Design review of the part built by this model. Coordinates are the model's own, in mm. A direction names the side the tool comes from. Coordinates: 2 decimals unless noted, no trailing zeros. Write each loop counter-clockwise with the first axis right and the second up, starting at its lowest first coordinate (ties: lowest second). Pieces come first, ordered by that corner, then holes. Notation, with made-up numbers: M -10,23.5 L 8,23.5 A26 ccw 8,39.5 Z; hole C -27,-4 d2. An arc over 180 degrees is marked long. Write item = value, one per line.
Autodesk Inventor part; units mm, degrees
ref_plane "YZ Plane" through (0, 0, 0) normal (1, 0, 0) x (0, 1, 0)
ref_plane "XZ Plane" through (0, 0, 0) normal (0, 1, 0) x (-1, 0, 0)
ref_plane "XY Plane" through (0, 0, 0) normal (0, 0, 1) x (1, 0, 0)
sketch "Sketch1" plane through (0, 0, 0) normal (0, 0, 1) x (1, 0, 0)
  circle A0 centre (0, 0) radius 24.5
  dimension "d0" = 49
extrude "Extrusion1" add sketch "Sketch1" along normal blind 83
sketch "Sketch2" plane through (0, 0, 0) normal (0, 0, 1) x (1, 0, 0)
  circle A0 centre (0, 0) radius 3
  dimension "d3" = 6
extrude "Extrusion2" add sketch "Sketch2" against normal blind 20
chamfer "Chamfer1" distance 3 distance2 8 1 edges at (-24.5, 0, 0) measured on face at (17.067, -2.1937, 0)
sketch "Sketch4" plane through (0, 0, 83) normal (0, 0, 1) x (1, 0, 0)
  circle A0 centre (0, 0) radius 7.25
  circle A1 centre (0, 0) radius 24.5
  dimension "d10" = 14.5
extrude "Extrusion3" cut sketch "Sketch4" against normal blind 5
chamfer "Chamfer2" distance 8.41 angle 45 1 edges at (-24.5, 0, 78)
properties part number "Motor SK3 5065 275KV"
Q1. For P1, Ø1, axis at x = -8.5, z = 72.5, coming from the +Y side; P2, Ø6, axis at y = 15.5, z = 52.5, coming from the +X side; P3, Ø1, axis at x = 16.5, z = 21, coming from the +Y side; P4, Ø16, axis at x = -7.5, y = -6.5, coming from the +Z side, all flat-tipped, find the tip position at first contact; note any pin that passes through.
Check result:
P1 = 20.43
P2 = 21.07
P3 = 18.55
P4 = 83
Q2. Consider section A-A, the plane y = 0. State the section outline as (x, z) points, and give its area (3 significant figures).
Check result:
outline = M -24.5,8 L -21.5,0 L -3,0 L -3,-20 L 3,-20 L 3,0 L 21.5,0 L 24.5,8 L 24.5,69.59 L 16.09,78 L 7.25,78 L 7.25,83 L -7.25,83 L -7.25,78 L -16.09,78 L -24.5,69.59 Z
area = 3,920 mm²
Q3. Wall thickness on line 1 (Z direction, x = 3, y = 12.5); line 2 (Y direction, x = 18.5, z = 27.5); line 3 (Z direction, x = 3.5, y = -16): over which ranges is each line inside the solid? List them lowest first.
Check result:
line_1 = 0 to 78
line_2 = -16.06 to 16.06
line_3 = 0 to 77.71
Q4. Machinability: for faces 1 (the cylindrical face through (3.35, -6.43, 80.54)), 2 (the flat face through (0, 0, 83)), 3 (the cylindrical face through (-3, 0, -10)), which of the approach directions +Z, -Z, +X, -X, +Y, -Y give a long, thin tool a straight path to every point of the face, cutting with its end or side? Answer none if there is none.
Check result:
face_1 = +Z
face_2 = +Z, +X, -X, +Y, -Y
face_3 = -Z
Q5. Consider section C-C, the plane z = 54. State the section outline as (x, y) points.
Check result:
outline = C 0,0 d49
